CAD build for the part. Positions are in the model's coordinates, mm. Give positions to 0.01 mm unless a question says otherwise; leave off trailing zeros. Loops run counter-clockwise (first coordinate to the right, second up) from the corner with the lowest first, then second, coordinate; pieces in that order, holes last. Notation, with made-up numbers: M 63,-25.75 L 68,-25.75 A24 cw 68,13.25 Z; hole C 45,-38.75 d3. An arc over 180 degrees is marked long. Answer as CSV lines item,"result".
```python
from build123d import *

# Parameters (mm, degrees)
SKETCH2_W                 = 47.5
SKETCH2_H                 = 35
BOSS_EXTRUDE1_DEPTH       = 3
F_3_0MM_DOWEL_HOLE1_D     = 3
F_3_0MM_DOWEL_HOLE1_DEPTH = 3
CUT_EXTRUDE1_REACH        = 5
SKETCH5_W                 = 47.5
SKETCH5_H                 = 11


with BuildPart() as part:
    # Sketch2 → Boss-Extrude1 (new body)
    with BuildSketch(Plane(origin=(0, 0, 0), x_dir=(1, 0, 0), z_dir=(0, 1, 0))):
        with Locations((23.75, 17.5)):
            Rectangle(SKETCH2_W, SKETCH2_H)
    extrude(amount=BOSS_EXTRUDE1_DEPTH)

    # Ø3.0mm Dowel Hole1
    with Locations(Plane(origin=(0, 3, 0), x_dir=(1, 0, 0), z_dir=(0, 1, 0))):
        with Locations((5, 17.5), (42.5, 17.5)):
            Hole(F_3_0MM_DOWEL_HOLE1_D / 2, depth=F_3_0MM_DOWEL_HOLE1_DEPTH)

    # Sketch5 → Cut-Extrude1 (cut, up to next)
    with BuildSketch(Plane(origin=(0, 3, 0), x_dir=(1, 0, 0), z_dir=(0, 1, 0)), mode=Mode.PRIVATE) as cut_extrude1_sk1:
        with Locations((23.75, 29.5)):
            Rectangle(SKETCH5_W, SKETCH5_H)
    cut_extrude1_tool1 = extrude(cut_extrude1_sk1.sketch, amount=-CUT_EXTRUDE1_REACH, mode=Mode.PRIVATE) & part.part
    add(cut_extrude1_tool1.solids().sort_by_distance((23.75, 3, -29.5))[0], mode=Mode.SUBTRACT)


solid = part.part
```
Q1. Cut at B-B (x = 42.5). Write the cut outline in (y, z), and give its area (3 significant figures).
Solution:
outline,"M 0,-24 L 3,-24 L 3,-19 L 0,-19 Z; M 0,-16 L 3,-16 L 3,0 L 0,0 Z"
area,"63.0 mm²"
Q2. Mould opens along Z. For faces 1 (the flat face through (23, 1, 0)), 2 (the cylindrical face through (44, 1.48, -17.57)), 3 (the flat face through (23, 2, -24)) say: released by +Z, released by -Z, zero draft, split by the parting line, or undercut.
Solution:
face 1,"released by +Z"
face 2,"undercut"
face 3,"released by -Z"
Q3. Pin check, flat tip, straight feed: P1, Ø1.8, axis at x = 5, z = -17.5, coming from the +Y side. Stop position of the tip, or through.
Solution:
P1,"passes through"
Q4. Cut at C-C (x = 4.5). Write the cut outline in (y, z), and give its area (3 significant figures).
Solution:
outline,"M 0,-24 L 3,-24 L 3,-18.91 L 0,-18.91 Z; M 0,-16.09 L 3,-16.09 L 3,0 L 0,0 Z"
area,"63.5 mm²"
Q5. Cut at A-A (z = -17.5). Write the cut outline in (x, y), and give its area (4 significant figures).
Solution:
outline,"M 0,0 L 3.5,0 L 3.5,3 L 0,3 Z; M 6.5,0 L 41,0 L 41,3 L 6.5,3 Z; M 44,0 L 47.5,0 L 47.5,3 L 44,3 Z"
area,"124.5 mm²"
Q6. Wall check: line 1 (X direction, y = 2.25, z = -17.5); line 2 (Z direction, x = 42.5, y = 2.15); line 3 (Z direction, x = 6, y = 1.5). Give the ranges that are in metal, low to high. Write a range as [from, to].
Solution:
line 1,"x = [0, 3.5], [6.5, 41], [44, 47.5]"
line 2,"z = [-24, -19], [-16, 0]"
line 3,"z = [-24, -18.62], [-16.38, 0]"
